Geometry: see drawing. Coordinates: mm, zero at the bounding-box minimum. Coordinates: 2 decimals unless noted, no trailing zeros. Write each loop counter-clockwise with the first axis right and the second up, starting at its lowest first coordinate (ties: lowest second). Pieces come first, ordered by that corner, then holes.
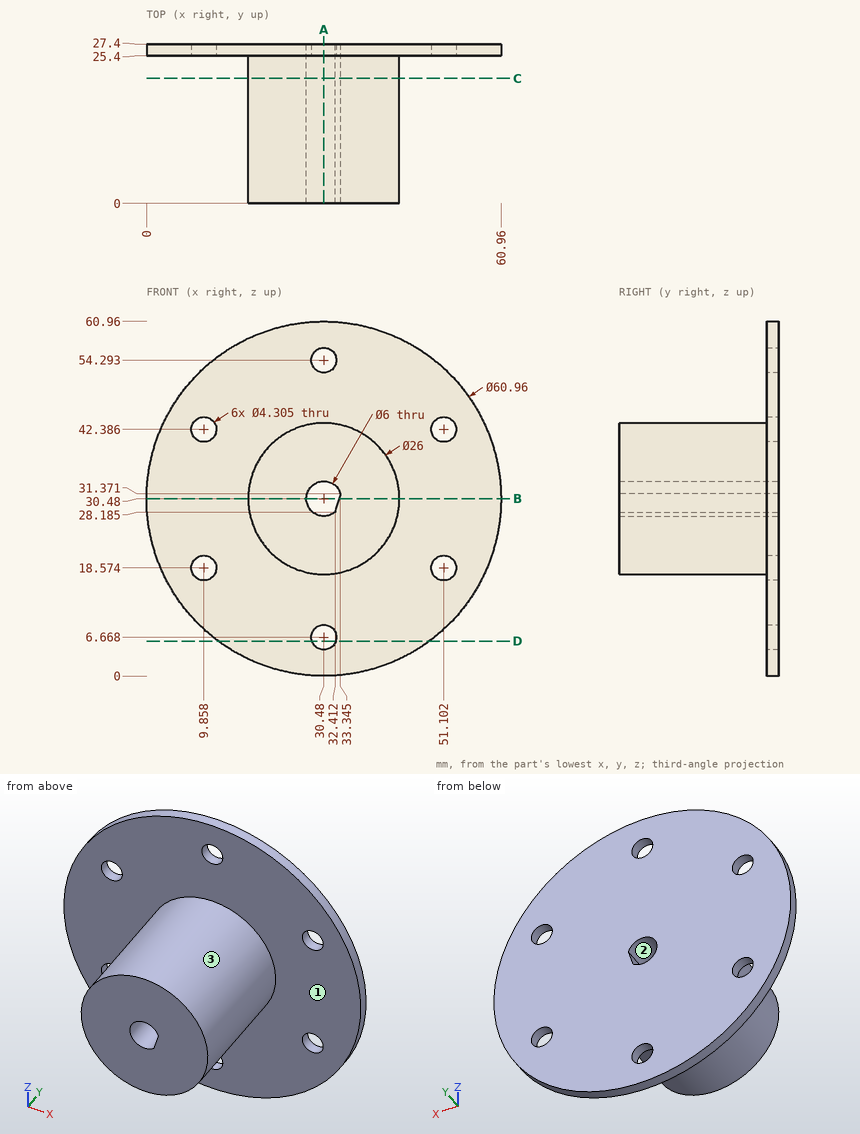
Item 1: Section D-D, the plane z = 6. Output: boundary loops of the cut face in (x, y).
Derived:
outline: (12.32, 25.4) - (28.43, 25.4) - (28.43, 27.4) - (12.32, 27.4) - close; (32.53, 25.4) - (48.64, 25.4) - (48.64, 27.4) - (32.53, 27.4) - close
Item 2: Section C-C, the plane y = 21.5. Output: boundary loops of the cut face in (x, z) (1 decimal), plus the area to 3 significant figures.
Derived:
outline: circle Ø26 at (30.5, 30.5); hole (32.4, 28.2) - (33.3, 31.4) arc R3 ccw (long way) to start
area: 504 mm2
Item 3: Pull-direction query (X, two-part tool) for the marked faces 1, 2 and 3; classes: released by +X, released by -X, zero draft, split by the parting line, or undercut.
Derived:
face 1: zero draft
face 2: undercut
face 3: split by the parting line
Item 4: Material intervals for probe 1 along Y at (x, z) = (51.5, 14.5); probe 2 along Z at (x, y) = (28, 26) (1 decimal); probe 3 along Z at (x, y) = (22.5, 3.25) (1 decimal), sorted ascending.
Derived:
probe 1: y = 25.4 to 27.4
probe 2: z = 0.1 to 28.8, 32.2 to 60.9
probe 3: z = 20.2 to 40.7
Item 5: Section B-B, the plane z = 30.48. Output: boundary loops of the cut face in (x, y), plus the area to 3 significant figures.
Derived:
outline: (0, 25.4) - (17.48, 25.4) - (17.48, 0) - (27.48, 0) - (27.48, 27.4) - (0, 27.4) - close; (33.08, 0) - (43.48, 0) - (43.48, 25.4) - (60.96, 25.4) - (60.96, 27.4) - (33.08, 27.4) - close
area: 629 mm2
Item 6: Section A-A, the plane x = 30.48. Output: boundary loops of the cut face in (y, z) (1 decimal).
Derived:
outline: (0, 17.5) - (25.4, 17.5) - (25.4, 8.8) - (27.4, 8.8) - (27.4, 27.5) - (0, 27.5) - close; (0, 33.5) - (27.4, 33.5) - (27.4, 52.1) - (25.4, 52.1) - (25.4, 43.5) - (0, 43.5) - close; (25.4, 0) - (27.4, 0) - (27.4, 4.5) - (25.4, 4.5) - close; (25.4, 56.4) - (27.4, 56.4) - (27.4, 61) - (25.4, 61) - close
Item 7: Pin query (flat end, axial travel): pin 1 (4 mm diameter, centred on x = 38, y = 12.5, fed in from +Z); pin 2 (1.5 mm diameter, centred on y = 18.5, z = 36.5, fed in from +X) (1 decimal); pin 3 (7 mm diameter, centred on x = 30.48, z = 54.29, fed in from -Y); pin 4 (3.5 mm diameter, centred on x = 9.86, z = 42.39, fed in from +Y). Return the tip coordinate at first contact, or that it passes through.
Derived:
pin 1: stops at z = 42.25
pin 2: stops at x = 42.4
pin 3: stops at y = 25.4
pin 4: passes through
